Geometry: final body of the model. Coordinates: model frame, mm. A direction names the side the tool comes from. Round coordinates to 2 decimals unless told otherwise and drop trailing zeros. Order: outer loops, then holes, each group sorted by start corner. A loop starts at its lowest first (then second) coordinate and runs counter-clockwise, first axis right, second up. Notation, with made-up numbers: (76, 39.5) -> (102, 39.5) arc R22 ccw to (102, 52.5) -> close; hole circle Ø10 at (55, 79.25). An arc over 180 degrees is marked (long way). Put each result on its own line as item: value.
```python
from build123d import *

# Parameters (mm, degrees)
F0_W      = 82.55
F0_H      = 34.925
F0_R      = 2.8702
F1_DEPTH  = 5.08
F4_R      = 1.27
F5_W      = 17.59966
F5_H      = 1.27
F5_W_2    = 9.99998
F6_DEPTH  = 3.556
F7_R      = 4.1275
F7_R_2    = 2.8702
F8_DEPTH  = 2.54
F9_W      = 18.00098
F9_H      = 1.27
F9_W_2    = 25.3492
F10_DEPTH = 5.08


with BuildPart() as f1:
    # F0 (on Top) → F1 (new body)
    with BuildSketch(Plane.XY):
        Rectangle(F0_W, F0_H)
        with Locations((35.75, -13)):
            Circle(F0_R, mode=Mode.SUBTRACT)
        with Locations((-36, 9.75)):
            Circle(F0_R, mode=Mode.SUBTRACT)
        with Locations((35.75, 10)):
            Circle(F0_R, mode=Mode.SUBTRACT)
    extrude(amount=F1_DEPTH)

    # F3: sweep along a path in F3_path
    with BuildLine(Plane(origin=(-41.275, 17.4625, 5.08), x_dir=(0, -1, 0), z_dir=(0, 0, -1))) as f3_path:
        Line((0, 0), (34.925, 0))
        Line((34.925, 0), (34.925, -82.55))
        Line((34.925, -82.55), (0, -82.55))
        Line((0, -82.55), (0, 0))
    # F2 (on Front) → F3 (sweep)
    with BuildSketch(Plane.XZ):
        with BuildLine():
            Line((-41.275, 0), (-41.275, 5.08))
            ThreePointArc((-41.275, 5.08), (-43.0710512242, 5.8239487758), (-43.815, 7.62))
            Line((-43.815, 7.62), (-43.815, 8.89))
            Line((-43.815, 8.89), (-46.355, 8.89))
            Line((-46.355, 8.89), (-46.355, 10.16))
            Line((-46.355, 10.16), (-48.895, 10.16))
            Line((-48.895, 10.16), (-48.895, 7.62))
            ThreePointArc((-48.895, 7.62), (-46.6631536726, 2.2318463274), (-41.275, 0))
        make_face()
    sweep(path=f3_path.line, transition=Transition.RIGHT)

    # F4
    f4_edges = [f1.edges().sort_by_distance(p)[0] for p in [
        (46.663154, 22.850654, 2.231846),
        (-46.663154, 22.850654, 2.231846),
        (-46.663154, -22.850654, 2.231846),
        (46.663154, -22.850654, 2.231846),
        (48.895, 25.0825, 8.89),
        (-48.895, 25.0825, 8.89),
        (-48.895, -25.0825, 8.89),
        (48.895, -25.0825, 8.89),
    ]]
    fillet(f4_edges, radius=F4_R)

    # F5 (on face) → F6 (cut)
    with BuildSketch(Plane(origin=(0, 25.0825, 0), x_dir=(-1, 0, 0), z_dir=(0, 1, 0))):
        with Locations((24.20069, 9.525)):
            Rectangle(F5_W, F5_H)
        with Locations((-22.33125, 9.525)):
            Rectangle(F5_W_2, F5_H)
    extrude(amount=-F6_DEPTH, mode=Mode.SUBTRACT)

    # F7 (on face) → F8 (join)
    with BuildSketch(Plane.XY.offset(5.08)):
        with Locations((-36, 9.75)):
            Circle(F7_R)
        with Locations((-36, 9.75)):
            Circle(F7_R_2, mode=Mode.SUBTRACT)
        with Locations((35.75, 10)):
            Circle(F7_R)
        with Locations((35.75, 10)):
            Circle(F7_R_2, mode=Mode.SUBTRACT)
        with Locations((35.75, -13)):
            Circle(F7_R)
        with Locations((35.75, -13)):
            Circle(F7_R_2, mode=Mode.SUBTRACT)
    extrude(amount=F8_DEPTH)

    # F9 (on face) → F10 (cut)
    with BuildSketch(Plane.XZ.offset(25.0825)):
        with Locations((11.99853, 9.525)):
            Rectangle(F9_W, F9_H)
        with Locations((-20.69422, 9.525)):
            Rectangle(F9_W_2, F9_H)
    extrude(amount=-F10_DEPTH, mode=Mode.SUBTRACT)


solid = f1.part
```
1. Draft query along X for faces 1 (the face through (-0.67, 22.91, 2.29)), 2 (the face through (0.613, -19.278, 5.844)), 3 (the face through (-48.895, 0, 9)), 4 (the face through (37, 13, 7.62)). Return one class per face: +X half, -X half, draft (parallel to the pull), parting line (faces both ways), or undercut.
Ans:
face 1: draft
face 2: undercut
face 3: -X half
face 4: undercut
2. Cut plane C-C on x = -36. Return loops of the section in (y, z), and give its area (3 significant figures).
Ans:
outline: (-25.08, 7.62) arc R7.62 ccw to (-17.46, 0) -> (6.88, 0) -> (6.88, 7.62) -> (5.62, 7.62) -> (5.62, 5.08) -> (-17.46, 5.08) arc R2.54 cw to (-20, 7.62) -> (-20, 8.89) -> (-22.54, 8.89) -> (-22.54, 10.16) -> (-25.08, 10.16) -> close; (12.62, 0) -> (17.46, 0) arc R7.62 ccw to (25.08, 7.62) -> (25.08, 10.16) -> (22.54, 10.16) -> (22.54, 8.89) -> (20, 8.89) -> (20, 7.62) arc R2.54 cw to (17.46, 5.08) -> (13.88, 5.08) -> (13.88, 7.62) -> (12.62, 7.62) -> close
area: 255 mm²
3. Set-up query: faces 5 (the face through (0.67, -22.91, 2.29)), 6 (the face through (-43.091, -0.28, 5.844)). Return all of +Z, -Z, +X, -X, +Y, -Y with unobstructed straight access to the full face (end or side cutting, diameter ignored); none if empty.
Ans:
face 5: -Z, +X, -X, -Y
face 6: +Z
4. Material intervals for probe 1 along X at (y, z) = (-2, 8.25) (3 decimals); probe 2 along Y at (x, z) = (35.5, 6); probe 3 along Y at (x, z) = (-35.5, 6.75), sorted ascending.
Ans:
probe 1: -48.895 to -43.815, 43.815 to 48.895
probe 2: -24.91 to -19.42, -17.12 to -15.86, -10.14 to -8.88, 5.88 to 7.14, 12.86 to 14.12, 19.42 to 24.91
probe 3: -25.03 to -19.85, 5.65 to 6.92, 12.58 to 13.85, 19.85 to 25.03
5. Cut plane B-B on x = 35.75. State how many separate pieces and enclosed holes the cut face has, and give its area (3 significant figures).
Ans:
separate pieces: 3
enclosed holes: 0
area: 232 mm²
6. Contact query for flat-ended pins moving along their axis: P1, Ø2.5, axis at x = 37.5, y = 10.5, coming from the +Z side; P2, Ø1.4, axis at y = -24.5, z = 9.5, coming from the +X side (3 decimals); P3, Ø5, axis at x = -10, z = 3.5, coming from the +Y side; P4, Ø25, axis at x = -1.5, y = -9, coming from the +Z side. Output: stop coordinate, or through.
Ans:
P1: z = 7.62
P2: x = 48.895
P3: y = 24.91
P4: z = 8.89
7. Cut plane D-D on y = -6.5. Return loops of the section in (x, z) (3 decimals).
Ans:
outline: (-48.895, 7.62) arc R7.62 ccw to (-41.275, 0) -> (41.275, 0) arc R7.62 ccw to (48.895, 7.62) -> (48.895, 10.16) -> (46.355, 10.16) -> (46.355, 8.89) -> (43.815, 8.89) -> (43.815, 7.62) arc R2.54 cw to (41.275, 5.08) -> (-41.275, 5.08) arc R2.54 cw to (-43.815, 7.62) -> (-43.815, 8.89) -> (-46.355, 8.89) -> (-46.355, 10.16) -> (-48.895, 10.16) -> close
8. Cut plane A-A on y = -13. Return loops of the section in (x, z) (1 decimal), and give its area (3 significant figures).
Ans:
outline: (-48.9, 7.6) arc R7.6 ccw to (-41.3, 0) -> (32.9, 0) -> (32.9, 7.6) -> (31.6, 7.6) -> (31.6, 5.1) -> (-41.3, 5.1) arc R2.5 cw to (-43.8, 7.6) -> (-43.8, 8.9) -> (-46.4, 8.9) -> (-46.4, 10.2) -> (-48.9, 10.2) -> close; (38.6, 0) -> (41.3, 0) arc R7.6 ccw to (48.9, 7.6) -> (48.9, 10.2) -> (46.4, 10.2) -> (46.4, 8.9) -> (43.8, 8.9) -> (43.8, 7.6) arc R2.5 cw to (41.3, 5.1) -> (39.9, 5.1) -> (39.9, 7.6) -> (38.6, 7.6) -> close
area: 497 mm²
